The model under review builds one solid part; all positions refer to its coordinate system, in mm. Give positions to 0.01 mm unless a question says otherwise; leave off trailing zeros. Write each loop counter-clockwise with the first axis right and the second up, starting at its lowest first coordinate (ties: lowest second). Pieces come first, ordered by that corner, then holes. Notation, with made-up numbers: (78.5, 29.5) -> (126.5, 29.5) arc R8 cw to (126.5, 43.5) -> close; hole circle Ø4 at (-3, 55). An arc over 180 degrees is marked (long way). Use CSV: the item, a comma, the result in double quotes.
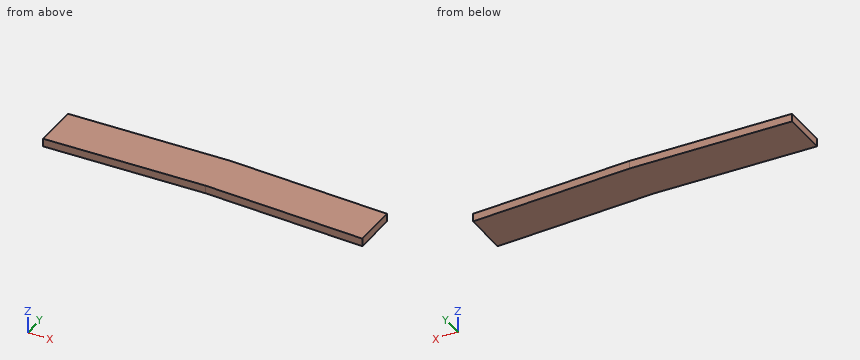
Autodesk Inventor part; units mm, degrees
ref_plane "YZ Plane" through (0, 0, 0) normal (1, 0, 0) x (0, 1, 0)
ref_plane "XZ Plane" through (0, 0, 0) normal (0, 1, 0) x (-1, 0, 0)
ref_plane "XY Plane" through (0, 0, 0) normal (0, 0, 1) x (1, 0, 0)
sketch "Sketch1" plane through (0, 0, 0) normal (0, 0, 1) x (1, 0, 0)
  line L0 (0, 0) -> (119, 0)
  line L1 (0, 0) -> (0, 16.6)
  line L2 (0, 0) -> (59.5, 0)
  line L3 (59.5, 2) -> (59.5, 18.5)
  line L4 (0, 16.6) -> (59.5, 18.5)
  line L5 (59.5, 2) -> (0, 0)
  line L6 (119, 0) -> (119, 16.5)
  line L7 (59.5, 18.5) -> (119, 16.5)
  line L8 (119, 0) -> (59.5, 2)
  dimension "d0" = 119
  dimension "d1" = 16.6
  dimension "d2" = 59.5
  dimension "d3" = 2
  dimension "d4" = 16.5
  dimension "d5" = 16.5
extrude "Extrusion1" add sketch "Sketch1" along normal blind 3 contours L1 L4 L3 L5 | L3 L7 L6 L8
properties part number "E"
Q1. To check wall thickness, follow probe 1 along Y at (x, z) = (77, 2.3); probe 2 along Y at (x, z) = (23, 2.6). State the ranges of each line that lie inside material, in increasing order.
Derived:
probe 1,"y = 1.41 to 17.91"
probe 2,"y = 0.77 to 17.33"
Q2. Consider section B-B (x = 36). Write out the cut boundary in (y, z).
Derived:
outline,"(1.21, 0) -> (17.75, 0) -> (17.75, 3) -> (1.21, 3) -> close"
Q3. Consider section A-A (z = 2.55). Write out the cut boundary in (x, y), then the cut area to 3 significant figures.
Derived:
outline,"(0, 0) -> (59.5, 2) -> (119, 0) -> (119, 16.5) -> (59.5, 18.5) -> (0, 16.6) -> close"
area,"1,970 mm2"
Q4. Insertion check: pin 1 (1 mm diameter, centred on x = 58.5, z = 1, fed in from +Y). The pin has a flat end and moves straight along its axis. Give the tip position at first contact, or say it passes through.
Derived:
pin 1,"stops at y = 18.48"
Q5. Consider section C-C (x = 20). Write out the cut boundary in (y, z), then the cut area to 3 significant figures.
Derived:
outline,"(0.67, 0) -> (17.24, 0) -> (17.24, 3) -> (0.67, 3) -> close"
area,"49.7 mm2"
